Source: CAD feature listing. Evaluate the final solid. Frame: model axes, mm. Face numbers are marked on the shaded views. A direction names the side the tool comes from. Round coordinates to 2 decimals unless told otherwise and drop trailing zeros. Write each loop counter-clockwise with the first axis right and the second up, starting at its lowest first coordinate (ties: lowest second). Pieces come first, ordered by that corner, then holes.
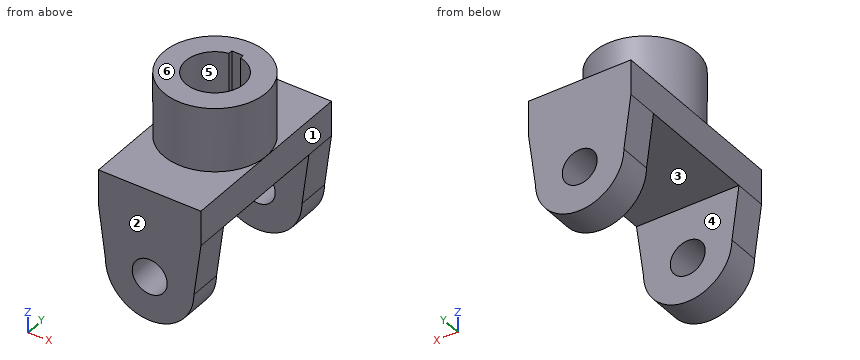
from build123d import *

# Parameters (mm, degrees)
SKETCH1_W           = 88
SKETCH1_H           = 162
BOSS_EXTRUDE1_DEPTH = 30
SKETCH2_R           = 44
BOSS_EXTRUDE2_DEPTH = 55
SKETCH3_R           = 15
BOSS_EXTRUDE3_DEPTH = 28


with BuildPart() as part:
    # Sketch1 → Boss-Extrude1 (new body)
    with BuildSketch(Plane.XY):
        Rectangle(SKETCH1_W, SKETCH1_H)
    extrude(amount=BOSS_EXTRUDE1_DEPTH)

    # Sketch2 → Boss-Extrude2 (add)
    with BuildSketch(Plane.XY.offset(30)):
        Circle(SKETCH2_R)
        with BuildLine():
            Line((-5, 24.494897428), (-5, 28))
            Line((-5, 28), (5, 28))
            Line((5, 28), (5, 24.494897428))
            ThreePointArc((5, 24.494897428), (0, -25), (-5, 24.494897428))
        make_face(mode=Mode.SUBTRACT)
    extrude(amount=BOSS_EXTRUDE2_DEPTH)

    # Sketch3 → Boss-Extrude3 (add)
    with BuildSketch(Plane.XZ.offset(81)):
        with BuildLine():
            Line((-44, 0), (-38, -45))
            ThreePointArc((-38, -45), (0, -83), (38, -45))
            Line((38, -45), (44, 0))
            Line((44, 0), (-44, 0))
        make_face()
        with Locations(Location((0, -45, 0), (0, 0, 270))):
            Circle(SKETCH3_R, mode=Mode.SUBTRACT)
    boss_extrude3 = extrude(amount=-BOSS_EXTRUDE3_DEPTH)

    # Mirror1: Boss-Extrude3 across plane
    add(boss_extrude3.mirror(Plane.ZX))


solid = part.part
1) Reachability of the marked faces 4, 5 and 6 from +Z, -Z, +X, -X, +Y, -Y: full face, straight path, thin tool, end or side. Return the list, or none.
Taken from the geometry:
face 4: -Z, +X, -X
face 5: +Z
face 6: +Z, +X, -X, +Y, -Y
2) Pull-direction query (Y, two-part tool) for the marked faces 1, 2 and 3; classes: released by +Y, released by -Y, zero draft, split by the parting line, or undercut.
Taken from the geometry:
face 1: zero draft
face 2: released by -Y
face 3: undercut
3) Material intervals for line 1 (Y direction, x = -14.5, z = -38.5); line 2 (Y direction, x = 0, z = 51); line 3 (X direction, y = -72, z = -45), sorted ascending.
Taken from the geometry:
line 1: y = -81 to -53, 53 to 81
line 2: y = -44 to -25, 28 to 44
line 3: x = -38 to -15, 15 to 38
4) Section query A-A on x = 0. Return the cut outline in (y, z).
Taken from the geometry:
outline: (-81, -83) - (-53, -83) - (-53, -60) - (-81, -60) - close; (-81, -30) - (-53, -30) - (-53, 0) - (53, 0) - (53, -30) - (81, -30) - (81, 30) - (44, 30) - (44, 85) - (28, 85) - (28, 30) - (-25, 30) - (-25, 85) - (-44, 85) - (-44, 30) - (-81, 30) - close; (53, -83) - (81, -83) - (81, -60) - (53, -60) - close
5) Section query D-D on y = -21. Return the cut outline in (x, z), then the cut area to 3 significant figures.
Taken from the geometry:
outline: (-44, 0) - (44, 0) - (44, 30) - (38.67, 30) - (38.67, 85) - (13.56, 85) - (13.56, 30) - (-13.56, 30) - (-13.56, 85) - (-38.67, 85) - (-38.67, 30) - (-44, 30) - close
area: 5,400 mm2
6) Section query C-C on z = 74.5. Return the cut outline in (x, y).
Taken from the geometry:
outline: circle Ø88 at (0, 0); hole (-5, 24.49) arc R25 ccw (long way) to (5, 24.49) - (5, 28) - (-5, 28) - close
7) Contact query for flat-ended pins moving along their axis: P1, Ø4, axis at y = 26.5, z = 45.5, coming from the +X side; P2, Ø3, axis at y = 26, z = 49, coming from the -X side; P3, Ø1.5, axis at x = 18, y = 14, coming from the -Z side. Output: stop coordinate, or through.
Taken from the geometry:
P1: stops at x = 36.55
P2: stops at x = -36.55
P3: stops at z = 0
8) Section query B-B on z = -42. Return the cut outline in (x, y), then the cut area to 3 significant figures.
Taken from the geometry:
outline: (-38.4, -81) - (-14.7, -81) - (-14.7, -53) - (-38.4, -53) - close; (-38.4, 53) - (-14.7, 53) - (-14.7, 81) - (-38.4, 81) - close; (14.7, -81) - (38.4, -81) - (38.4, -53) - (14.7, -53) - close; (14.7, 53) - (38.4, 53) - (38.4, 81) - (14.7, 81) - close
area: 2,650 mm2
